from build123d import *

# Parameters (mm, degrees)
SKETCH_R     = 16.55
PAD_DEPTH    = 6
SKETCH001_R  = 2
POCKET_DEPTH = 6.001
PAD001_DEPTH = 1


with BuildPart() as part:
    # Sketch → Pad (new body)
    with BuildSketch(Plane.XY):
        Circle(SKETCH_R)
    extrude(amount=PAD_DEPTH)

    # Sketch001 (on Face3 of Pad) → Pocket (cut, through all)
    with BuildSketch(Plane.XY.offset(6)):
        with Locations((0, 16.55)):
            Circle(SKETCH001_R)
    extrude(amount=-POCKET_DEPTH, mode=Mode.SUBTRACT)

    # Sketch002 (on Face4 of Pocket) → Pad001 (join)
    with BuildSketch(Plane.XY.offset(6)):
        with BuildLine():
            ThreePointArc((-1.996346, 18.442436), (0, -18.550171), (1.996346, 18.442436))
            Line((1.992658, 16.378788), (1.996346, 18.442436))
            ThreePointArc((-1.996346, 16.429154), (-0.025251, 14.550159), (1.992658, 16.378788))
            Line((-1.996346, 16.429154), (-1.996346, 18.442436))
        make_face()
    extrude(amount=PAD001_DEPTH)


solid = part.part
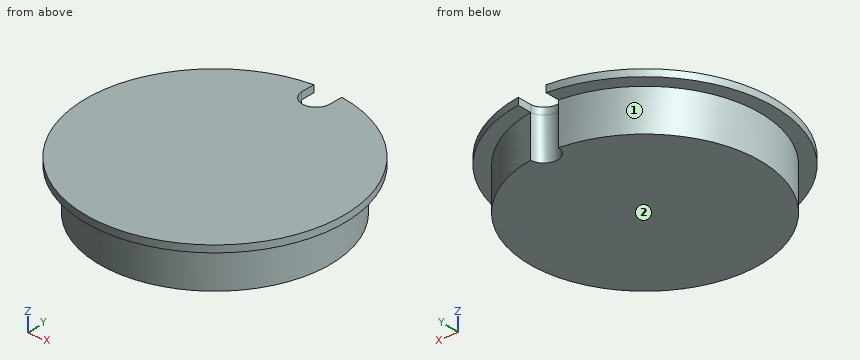
Design review of the part built by this model. Coordinates are the model's own, in mm. Face numbers are marked on the shaded views. A direction names the side the tool comes from. Give positions to 0.01 mm unless a question says otherwise; leave off trailing zeros. Loops run counter-clockwise (first coordinate to the right, second up) from the corner with the lowest first, then second, coordinate; pieces in that order, holes last. Notation, with made-up numbers: M -31,61 L 3,61 A21 cw 3,98 Z; hole C -14.75,19.25 d4. An arc over 180 degrees is marked long. One line per question, with ' | ' between items. Start each with the question number.
1. Add section B-B (x = 0). Write out the cut boundary in (y, z).
2. Add section C-C (z = 5.5). Write out the cut boundary in (x, y).
3. Insertion check: P1, Ø1.5, axis at x = -1.5, z = 5.5, coming from the -Y side; P2, Ø3, axis at y = -3.5, z = 3.5, coming from the -X side. Each pin has a flat end and moves straight along its axis. Give the tip position at first contact, or say it passes through.
4. Add section D-D (y = 10.5). Write out the cut boundary in (x, z).
5. For the marked faces 1 and 2, list the 3-axis set-ups (+Z, -Z, +X, -X, +Y, -Y) from which the entire face can be reached by the end or side of a thin tool; tool diameter is ignored.
6. Add section A-A (y = 0). Write out the cut boundary in (x, z).
7. To check wall thickness, follow L1, parallel to Z at x = 11.5, y = 12; L2, parallel to X at y = 0.5, z = 2.25; L3, parallel to Y at x = 4.5, z = 4. State the ranges of each line that lie inside material, in increasing order.
Worked out:
1) outline: M -18.55,6 L -16.55,6 L -16.55,0 L 14.55,0 L 14.55,7 L -18.55,7 Z
2) outline: M -2,16.43 A16.55 ccw long 2,16.43 A2 cw Z
3) P1: stops at y = -18.53 | P2: stops at x = -16.43
4) outline: M -15.29,6 L -12.79,6 L -12.79,0 L 12.79,0 L 12.79,6 L 15.29,6 L 15.29,7 L -15.29,7 Z
5) face 1: -Z | face 2: -Z, +X, -X, +Y, -Y
6) outline: M -18.55,6 L -16.55,6 L -16.55,0 L 16.55,0 L 16.55,6 L 18.55,6 L 18.55,7 L -18.55,7 Z
7) L1: z = 6 to 7 | L2: x = -16.54 to 16.54 | L3: y = -15.93 to 15.93
